from build123d import *

# Parameters (mm, degrees)
F0_R     = 35
F1_DEPTH = 228


with BuildPart() as f1:
    # F0 (on Top) → F1 (new body)
    with BuildSketch(Plane.XY):
        with BuildLine():
            ThreePointArc((-92.70522, 37.493228), (0, -100), (92.70522, 37.493228))
            ThreePointArc((92.70522, 37.493228), (90.589498, 50.828634), (94.536024, 63.741197))
            Line((94.536024, 63.741197), (143.30127, 148.205081))
            Line((143.30127, 148.205081), (56.69873, 198.205081))
            Line((56.69873, 198.205081), (8.660254, 115))
            ThreePointArc((8.660254, 115), (0, 110), (-8.660254, 115))
            Line((-8.660254, 115), (-56.69873, 198.205081))
            Line((-56.69873, 198.205081), (-143.30127, 148.205081))
            Line((-143.30127, 148.205081), (-94.536024, 63.741197))
            ThreePointArc((-94.536024, 63.741197), (-90.589498, 50.828634), (-92.70522, 37.493228))
        make_face()
        Circle(F0_R, mode=Mode.SUBTRACT)
    extrude(amount=F1_DEPTH)


solid = f1.part
Verification items for the finished model (mm, model axes). A direction names the side the tool comes from. Coordinates: 2 decimals unless noted, no trailing zeros. Order: outer loops, then holes, each group sorted by start corner. A loop starts at its lowest first (then second) coordinate and runs counter-clockwise, first axis right, second up. Notation, with made-up numbers: M -31,85 L 25,85 A19 cw 25,118 Z; hole C 89,22 d3. An arc over 180 degrees is marked long. Return JSON: item names as keys, results as strings.
1) Thickness scan on L1, parallel to X at y = 48, z = 14.5; L2, parallel to Y at x = -1.5, z = 200; L3, parallel to X at y = -26, z = 187.5. Record the ranges inside material, lowest first. Write a range as [from, to].
Answer list:
{"L1": "[-90.53, 90.53]", "L2": "[-99.99, -34.97], [34.97, 110.11]", "L3": "[-96.56, -23.43], [23.43, 96.56]"}
2) Cross-section at A-A, the plane x = 0. Record the boundary of the cut face in (y, z).
Answer list:
{"outline": "M -100,0 L -35,0 L -35,228 L -100,228 Z; M 35,0 L 110,0 L 110,228 L 35,228 Z"}
3) Cross-section at B-B, the plane y = 0. Record the boundary of the cut face in (x, z), and give its area (3 significant figures).
Answer list:
{"outline": "M -100,0 L -35,0 L -35,228 L -100,228 Z; M 35,0 L 100,0 L 100,228 L 35,228 Z", "area": "29,600 mm2"}
4) Gauge pin test, flat ends, axial feed: pin 1 (1 mm diameter, centred on y = 24.5, z = 173.5, fed in from -X); pin 2 (4 mm diameter, centred on x = -8.5, z = 153, fed in from +Y); pin 3 (2 mm diameter, centred on y = 99, z = 154, fed in from +X). Record the tip position at first contact, or that the pin passes through.
Answer list:
{"pin 1": "x = -97.08", "pin 2": "y = 118.19", "pin 3": "x = 115.47"}
5) Release check for a two-part mould opening along Y. For faces 1 (the flat face through (-99.394, 173.555, 112.404)), 2 (the flat face through (-2, 51, 0)), 3 (the cylindrical face through (-90.6, 51, 112.4)), 4 (the cylindrical face through (-2.737, -99.963, 112.404)) record: +Y half, -Y half, draft (parallel to the pull), parting line (faces both ways), or undercut.
Answer list:
{"face 1": "+Y half", "face 2": "draft", "face 3": "undercut", "face 4": "undercut"}
6) Cross-section at C-C, the plane z = 204.5. Record the boundary of the cut face in (x, y), and give its area (3 significant figures).
Answer list:
{"outline": "M -143.3,148.21 L -94.54,63.74 A30 cw -92.71,37.49 A100 ccw long 92.71,37.49 A30 cw 94.54,63.74 L 143.3,148.21 L 56.7,198.21 L 8.66,115 A10 cw -8.66,115 L -56.7,198.21 Z; hole C 0,0 d70", "area": "48,600 mm2"}
7) Access from +Z, -Z, +X, -X, +Y, -Y to the whole of each face (thin tool, end or side, straight path). Record for faces 5 (the flat face through (100.606, 172.855, 112.404)), 6 (the flat face through (33.016, 157.185, 112.404)).
Answer list:
{"face 5": "+Z, -Z, +X, +Y", "face 6": "+Z, -Z, +Y"}
8) Cross-section at D-D, the plane y = -80. Record the boundary of the cut face in (x, z).
Answer list:
{"outline": "M -60,0 L 60,0 L 60,228 L -60,228 Z"}
